Here's how the part is built. I have some questions about the finished solid (model axes, mm). A direction names the side the tool comes from. Give positions to 0.01 mm unless a question says otherwise; leave off trailing zeros. Order: outer loops, then holes, each group sorted by start corner. A loop starts at its lowest first (then second) coordinate and runs counter-clockwise, first axis right, second up. Notation, with made-up numbers: M 84.25,31.25 L 96.25,31.25 A18 ccw 96.25,37.25 Z; hole C 20.5,87 d11. An arc over 180 degrees is marked long. One line per item, written item: value. Start each with the question number.
from build123d import *

# Parameters (mm, degrees)
SKETCH1_R           = 31.75
BOSS_EXTRUDE1_DEPTH = 3.175
SKETCH2_R           = 1.5875
CUT_EXTRUDE1_DEPTH  = 46.01339384
SKETCH6_R           = 7.332348419
BOSS_EXTRUDE2_DEPTH = 3.175
CUT_EXTRUDE2_DEPTH  = 46.01339384


with BuildPart() as part:
    # Sketch1 → Boss-Extrude1 (new body)
    with BuildSketch(Plane(origin=(0, 0, 0), x_dir=(1, 0, 0), z_dir=(0, 1, 0))):
        with Locations(Location((0, 0, 0), (0, 0, 270))):
            Circle(SKETCH1_R)
    extrude(amount=BOSS_EXTRUDE1_DEPTH)

    # Sketch2 → Cut-Revolve1 (revolve, cut)
    with BuildSketch(Plane.XY, mode=Mode.PRIVATE) as cut_revolve1_sk:
        with Locations((-31.75, 1.5875)):
            Circle(SKETCH2_R)
    revolve(cut_revolve1_sk.sketch.rotate(Axis((0, 0, 0), (0, 1, 0)), 270), axis=Axis((0, 0, 0), (0, 1, 0)), mode=Mode.SUBTRACT)

    # Sketch5 → Cut-Extrude1 (cut, through all)
    with BuildSketch(Plane(origin=(0, 3.175, 0), x_dir=(1, 0, 0), z_dir=(0, 1, 0))):
        with BuildLine():
            ThreePointArc((-23.660280874, -5.212986442), (-16.648813235, 1.003322249), (-7.332348419, 0))
            ThreePointArc((-7.332348419, 0), (-7.904270057, 10.91410008), (-18.107373639, 14.830903904))
            Line((-18.107373639, 14.830903904), (-26.67, 0))
            Line((-26.67, 0), (-23.660280874, -5.212986442))
        make_face()
        with BuildLine():
            ThreePointArc((-7.315561749, -23.096897519), (-9.193309174, -13.91663408), (-3.666174209, -6.35))
            ThreePointArc((-3.666174209, -6.35), (-13.404022957, -1.388248628), (-21.897626361, -8.265993615))
            Line((-21.897626361, -8.265993615), (-13.335, -23.096897519))
            Line((-13.335, -23.096897519), (-7.315561749, -23.096897519))
        make_face()
        with BuildLine():
            ThreePointArc((16.344719126, -17.883911077), (7.455504061, -14.919956329), (3.666174209, -6.35))
            ThreePointArc((3.666174209, -6.35), (-5.4997529, -12.302348707), (-3.790252722, -23.096897519))
            Line((-3.790252722, -23.096897519), (13.335, -23.096897519))
            Line((13.335, -23.096897519), (16.344719126, -17.883911077))
        make_face()
        with BuildLine():
            ThreePointArc((23.660280874, 5.212986442), (16.648813235, -1.003322249), (7.332348419, 0))
            ThreePointArc((7.332348419, 0), (7.904270057, -10.91410008), (18.107373639, -14.830903904))
            Line((18.107373639, -14.830903904), (26.67, 0))
            Line((26.67, 0), (23.660280874, 5.212986442))
        make_face()
        with BuildLine():
            ThreePointArc((7.315561749, 23.096897519), (9.193309174, 13.91663408), (3.666174209, 6.35))
            ThreePointArc((3.666174209, 6.35), (13.404022957, 1.388248628), (21.897626361, 8.265993615))
            Line((21.897626361, 8.265993615), (13.335, 23.096897519))
            Line((13.335, 23.096897519), (7.315561749, 23.096897519))
        make_face()
        with BuildLine():
            ThreePointArc((-16.344719126, 17.883911077), (-7.455504061, 14.919956329), (-3.666174209, 6.35))
            ThreePointArc((-3.666174209, 6.35), (5.4997529, 12.302348707), (3.790252722, 23.096897519))
            Line((3.790252722, 23.096897519), (-13.335, 23.096897519))
            Line((-13.335, 23.096897519), (-16.344719126, 17.883911077))
        make_face()
        with BuildLine():
            ThreePointArc((-21.044544984, 16.383407045), (-18.775429284, 17.386729294), (-16.344719126, 17.883911077))
            Line((-16.344719126, 17.883911077), (-13.335, 23.096897519))
            ThreePointArc((-13.335, 23.096897519), (-17.514451659, 20.113002836), (-21.044544984, 16.383407045))
        make_face()
        with BuildLine():
            Line((-13.335, 23.096897519), (3.790252722, 23.096897519))
            ThreePointArc((3.790252722, 23.096897519), (0.414884128, 25.549334154), (-3.666174209, 26.41681409))
            ThreePointArc((-3.666174209, 26.41681409), (-8.661145573, 25.224461488), (-13.335, 23.096897519))
        make_face()
        with BuildLine():
            ThreePointArc((3.666174209, 26.41681409), (5.669634616, 24.953363374), (7.315561749, 23.096897519))
            Line((7.315561749, 23.096897519), (13.335, 23.096897519))
            ThreePointArc((13.335, 23.096897519), (8.661145573, 25.224461488), (3.666174209, 26.41681409))
        make_face()
        with BuildLine():
            Line((13.335, 23.096897519), (21.897626361, 8.265993615))
            ThreePointArc((21.897626361, 8.265993615), (22.333814492, 12.415366882), (21.044544984, 16.383407045))
            ThreePointArc((21.044544984, 16.383407045), (17.514451659, 20.113002836), (13.335, 23.096897519))
        make_face()
        with BuildLine():
            ThreePointArc((24.710719194, 10.033407045), (24.4450639, 7.56663408), (23.660280874, 5.212986442))
            Line((23.660280874, 5.212986442), (26.67, 0))
            ThreePointArc((26.67, 0), (26.175597232, 5.111458652), (24.710719194, 10.033407045))
        make_face()
        with BuildLine():
            ThreePointArc((21.044544984, -16.383407045), (18.775429284, -17.386729294), (16.344719126, -17.883911077))
            Line((16.344719126, -17.883911077), (13.335, -23.096897519))
            ThreePointArc((13.335, -23.096897519), (17.514451659, -20.113002836), (21.044544984, -16.383407045))
        make_face()
        with BuildLine():
            Line((13.335, -23.096897519), (-3.790252722, -23.096897519))
            ThreePointArc((-3.790252722, -23.096897519), (-0.414884128, -25.549334154), (3.666174209, -26.41681409))
            ThreePointArc((3.666174209, -26.41681409), (8.661145573, -25.224461488), (13.335, -23.096897519))
        make_face()
        with BuildLine():
            ThreePointArc((-3.666174209, -26.41681409), (-5.669634616, -24.953363374), (-7.315561749, -23.096897519))
            Line((-7.315561749, -23.096897519), (-13.335, -23.096897519))
            ThreePointArc((-13.335, -23.096897519), (-8.661145573, -25.224461488), (-3.666174209, -26.41681409))
        make_face()
        with BuildLine():
            Line((-13.335, -23.096897519), (-21.897626361, -8.265993615))
            ThreePointArc((-21.897626361, -8.265993615), (-22.333814492, -12.415366882), (-21.044544984, -16.383407045))
            ThreePointArc((-21.044544984, -16.383407045), (-17.514451659, -20.113002836), (-13.335, -23.096897519))
        make_face()
        with BuildLine():
            ThreePointArc((-24.710719194, -10.033407045), (-24.4450639, -7.56663408), (-23.660280874, -5.212986442))
            Line((-23.660280874, -5.212986442), (-26.67, 0))
            ThreePointArc((-26.67, 0), (-26.175597232, -5.111458652), (-24.710719194, -10.033407045))
        make_face()
        with BuildLine():
            Line((-26.67, 0), (-18.107373639, 14.830903904))
            ThreePointArc((-18.107373639, 14.830903904), (-21.918930363, 13.133967272), (-24.710719194, 10.033407045))
            ThreePointArc((-24.710719194, 10.033407045), (-26.175597232, 5.111458652), (-26.67, 0))
        make_face()
        with BuildLine():
            Line((26.67, 0), (18.107373639, -14.830903904))
            ThreePointArc((18.107373639, -14.830903904), (21.918930363, -13.133967272), (24.710719194, -10.033407045))
            ThreePointArc((24.710719194, -10.033407045), (26.175597232, -5.111458652), (26.67, 0))
        make_face()
    extrude(amount=-CUT_EXTRUDE1_DEPTH, mode=Mode.SUBTRACT)

    # Sketch6 → Boss-Extrude2 (add)
    with BuildSketch(Plane(origin=(0, 3.175, 0), x_dir=(1, 0, 0), z_dir=(0, 1, 0))):
        Circle(SKETCH6_R)
    extrude(amount=-BOSS_EXTRUDE2_DEPTH)

    # Sketch7 → Cut-Extrude2 (cut, through all)
    with BuildSketch(Plane(origin=(0, 3.175, 0), x_dir=(1, 0, 0), z_dir=(0, 1, 0))):
        with BuildLine():
            Line((0.75, 1.299038106), (0.75, -1.299038106))
            ThreePointArc((0.75, -1.299038106), (-1.5, 0), (0.75, 1.299038106))
        make_face()
    extrude(amount=-CUT_EXTRUDE2_DEPTH, mode=Mode.SUBTRACT)


solid = part.part
Item 1: We'd pull the mould along Z, two halves only. Please class faces 1 (the face through (-5.42, 1.61, 4.94)), 2 (the face through (0, 0, 7)): +Z half, -Z half, draft (parallel to the pull), parting line (faces both ways), or undercut.
Item 2: For faces 3 (the face through (0, 3.175, 7)), 4 (the face through (0.75, 2, 0)), which set-ups out of +Z, -Z, +X, -X, +Y, -Y let a thin tool reach every point of the face, with its end or its side?
Item 3: I want a section at A-A on x = 12. Count the separate pieces of the cut face and the enclosed holes in it, plus the area to 3 significant figures.
Item 4: Please list where these lines run through material, in increasing order: probe 1 along Z at (x, y) = (-8, 2.55); probe 2 along X at (y, z) = (2.5, -9.5); probe 3 along X at (y, z) = (0.65, 19). Write a range as [from, to].
Item 5: I want a section at B-B on y = 1.2. Write out the boundary of the cut face in (x, z) (3 decimals).
Item 6: Will this pin go through, and if not, where does the flat tip stop? P1, Ø1, axis at x = -22.5, y = 1.5, coming from the -Z side.
Answer below:
1. face 1: undercut
1. face 2: draft
2. face 3: +Z, -Z, +X, -X, +Y
2. face 4: +Y, -Y
3. separate pieces: 4
3. enclosed holes: 0
3. area: 46.2 mm²
4. probe 1: z = [-29.42, -25.44], [-15.39, -11.04], [-0.36, 2.33], [10.76, 22.01], [25.44, 29.42]
4. probe 2: x = [-28.93, -24.92], [-7.05, -4.1], [3.63, 7.19], [22.21, 24.7], [24.92, 28.93]
4. probe 3: x = [-23.82, -18.72], [-9.16, -6.02], [18.72, 23.82]
5. outline: C 0,0 d60.421; hole M -24.711,-10.033 A10.033 ccw -6.023,-4.182 A7.332 cw -7.332,0 A11.586 cw -24.711,10.033 A26.67 ccw Z; hole M -21.045,-16.383 A26.67 ccw -3.666,-26.417 A10.033 ccw 0.61,-7.307 A7.332 cw -3.666,-6.35 A11.586 cw Z; hole M -21.045,16.383 A10.033 ccw -6.633,3.125 A7.332 cw -3.666,6.35 A11.586 cw -3.666,26.417 A26.67 ccw Z; hole M -0.61,7.307 A7.332 cw 3.666,6.35 A11.586 cw 21.045,16.383 A26.67 ccw 3.666,26.417 A10.033 ccw Z; hole M 0.75,-1.299 L 0.75,1.299 A1.5 ccw long Z; hole M 3.666,-26.417 A26.67 ccw 21.045,-16.383 A10.033 ccw 6.633,-3.125 A7.332 cw 3.666,-6.35 A11.586 cw Z; hole M 6.023,4.182 A7.332 cw 7.332,0 A11.586 cw 24.711,-10.033 A26.67 ccw 24.711,10.033 A10.033 ccw Z
6. P1: stops at z = -20.64
